from build123d import *

# Parameters (mm, degrees)
SKETCH2_R           = 2.5
SKETCH2_W           = 4
SKETCH2_H           = 4
BOSS_EXTRUDE1_DEPTH = 200


with BuildPart() as part:
    # Sketch2 → Boss-Extrude1 (new body)
    with BuildSketch(Plane.XY):
        Polygon((-10.400071427, 9), (-5.25, 3.849928573), (-5.25, 0), (-5.25, -3.849928573), (-10.400071427, -9), (-13, -9), (-13, -4.85), (-15, -4.85), (-15, -9), (-15, -15), (-9, -15), (-4.85, -15), (-4.85, -13), (-9, -13), (-9, -10.400071427), (-3.849928573, -5.25), (0, -5.25), (3.849928573, -5.25), (9, -10.400071427), (9, -13), (4.85, -13), (4.85, -15), (9, -15), (15, -15), (15, -9), (15, -4.85), (13, -4.85), (13, -9), (10.400071427, -9), (5.25, -3.849928573), (5.25, 0), (5.25, 3.849928573), (10.400071427, 9), (13, 9), (13, 4.85), (15, 4.85), (15, 9), (15, 15), (9, 15), (4.85, 15), (4.85, 13), (9, 13), (9, 10.400071427), (3.849928573, 5.25), (0, 5.25), (-3.849928573, 5.25), (-9, 10.400071427), (-9, 13), (-4.85, 13), (-4.85, 15), (-9, 15), (-15, 15), (-15, 9), (-15, 4.85), (-13, 4.85), (-13, 9), align=None)
        Circle(SKETCH2_R, mode=Mode.SUBTRACT)
        with Locations((-12, 12)):
            Rectangle(SKETCH2_W, SKETCH2_H, mode=Mode.SUBTRACT)
        with Locations((12, 12)):
            Rectangle(SKETCH2_W, SKETCH2_H, mode=Mode.SUBTRACT)
        with Locations((12, -12)):
            Rectangle(SKETCH2_W, SKETCH2_H, mode=Mode.SUBTRACT)
        with Locations((-12, -12)):
            Rectangle(SKETCH2_W, SKETCH2_H, mode=Mode.SUBTRACT)
    extrude(amount=BOSS_EXTRUDE1_DEPTH)


solid = part.part
Verification items for the finished model (mm, model axes). A direction names the side the tool comes from. Coordinates: 2 decimals unless noted, no trailing zeros. Order: outer loops, then holes, each group sorted by start corner. A loop starts at its lowest first (then second) coordinate and runs counter-clockwise, first axis right, second up. Notation, with made-up numbers: (-7.5, 59) -> (1.5, 59) arc R24 ccw to (1.5, 70) -> close; hole circle Ø5 at (60, -22). An arc over 180 degrees is marked (long way). Put each result on its own line as item: value. Start each with the question number.
1. Go/stop test with flat-tipped pins: pin 1 Ø8.5 at (x, z) = (0.5, 53) entering from -Y; pin 2 Ø2.5 at (x, z) = (0.5, 94) entering from +Y; pin 3 Ø2 at (x, y) = (7.5, -2.5) entering from +Z. Record where each tip stops, or that it passes through.
2. Access from +Z, -Z, +X, -X, +Y, -Y to the whole of each face (thin tool, end or side, straight path). Record for faces 1 (the flat face through (13, -7, 99)), 2 (the flat face through (-5.25, 0, 99)), 3 (the flat face through (5.25, 0, 99)), 4 (the flat face through (0, 3, 200)), 5 (the flat face through (0, 5.25, 99)).
3. Material ranges on L1, parallel to Y at x = -11, z = 36.5; L2, parallel to Y at x = 0, z = 141.5, recorded low to high. Write a range as [from, to].
4. Mould release check, pull along Y, two halves, no side actions. Record for faces 6 (the flat face through (-10, 15, 99)), 7 (the flat face through (-15, 10, 99)), 8 (the flat face through (12, -10, 99)): released by +Y, released by -Y, zero draft, split by the parting line, or undercut.
5. Cross-section at C-C, the plane z = 155. Count the separate pieces of the cut face and the enclosed holes in it, then the cut area to 3 significant figures.
6. Cross-section at A-A, the plane y = 0. Record the boundary of the cut face in (x, z).
Computed:
1. pin 1: y = -6.15
1. pin 2: y = 5.25
1. pin 3: through
2. face 1: +Z, -Z
2. face 2: +Z, -Z, -X
2. face 3: +Z, -Z, +X
2. face 4: +Z, +X, -X, +Y, -Y
2. face 5: +Z, -Z, +Y
3. L1: [-15, -14], [-10, -9], [9, 10], [14, 15]
3. L2: [-5.25, -2.5], [2.5, 5.25]
4. face 6: released by +Y
4. face 7: zero draft
4. face 8: undercut
5. separate pieces: 1
5. enclosed holes: 5
5. area: 287 mm2
6. outline: (-5.25, 0) -> (-2.5, 0) -> (-2.5, 200) -> (-5.25, 200) -> close; (2.5, 0) -> (5.25, 0) -> (5.25, 200) -> (2.5, 200) -> close
